Part print with two shaded views. Sizes in mm from the minimum x, y, z corner. A direction names the side the tool comes from. Round coordinates to 2 decimals unless told otherwise and drop trailing zeros. Loops run counter-clockwise (first coordinate to the right, second up) from the corner with the lowest first, then second, coordinate; pieces in that order, holes last.
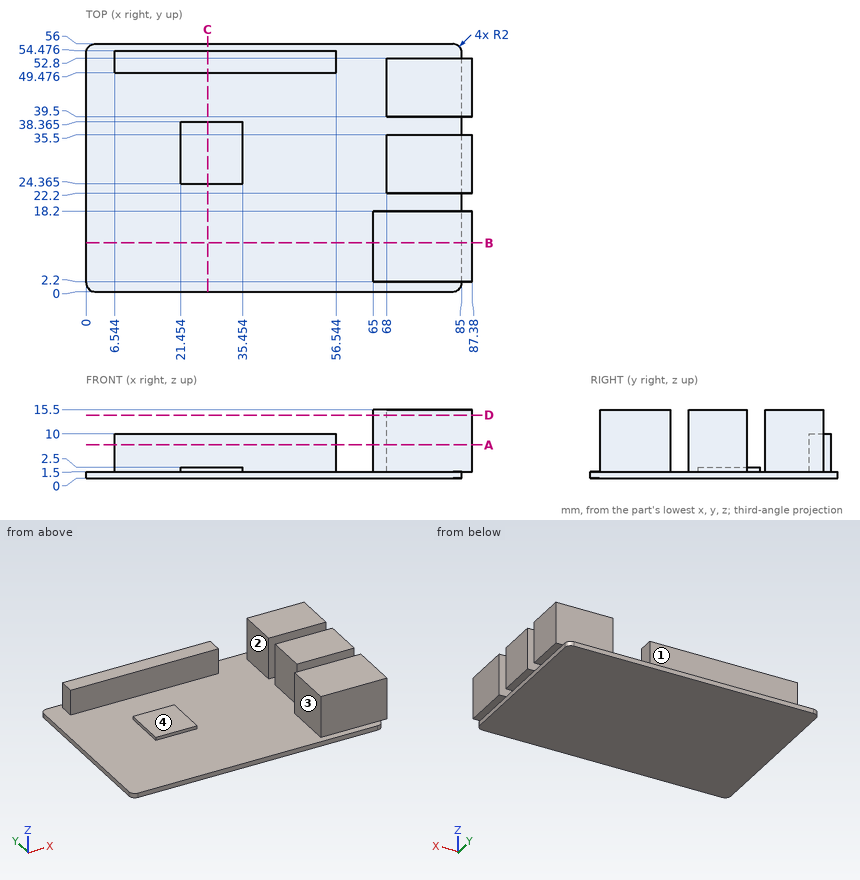
Item 1: Cut at A-A (z = 7.5). List the corners of the cut face in (x, y) (1 decimal).
Verdict:
outline: (6.5, 49.5) - (56.5, 49.5) - (56.5, 54.5) - (6.5, 54.5) - close; (65, 2.2) - (87.4, 2.2) - (87.4, 18.2) - (65, 18.2) - close; (68, 22.2) - (87.4, 22.2) - (87.4, 35.5) - (68, 35.5) - close; (68, 39.5) - (87.4, 39.5) - (87.4, 52.8) - (68, 52.8) - close
Item 2: Cut at C-C (x = 27.5). List the corners of the cut face in (y, z) (1 decimal).
Verdict:
outline: (0, 0) - (56, 0) - (56, 1.5) - (54.5, 1.5) - (54.5, 10) - (49.5, 10) - (49.5, 1.5) - (38.4, 1.5) - (38.4, 2.5) - (24.4, 2.5) - (24.4, 1.5) - (0, 1.5) - close
Item 3: Wall check: L1, parallel to Y at x = 73.5, z = 1.75; L2, parallel to X at y = 31, z = 1.75 (1 decimal); L3, parallel to Z at x = 48.5, y = 48.5. Give the ranges that are in metal, low to high.
Verdict:
L1: y = 2.2 to 18.2, 22.2 to 35.5, 39.5 to 52.8
L2: x = 21.5 to 35.5, 68 to 87.4
L3: z = 0 to 1.5
Item 4: Cut at D-D (z = 14.25). List the corners of the cut face in (x, y).
Verdict:
outline: (65, 2.2) - (87.38, 2.2) - (87.38, 18.2) - (65, 18.2) - close; (68, 22.2) - (87.38, 22.2) - (87.38, 35.5) - (68, 35.5) - close; (68, 39.5) - (87.38, 39.5) - (87.38, 52.8) - (68, 52.8) - close
Item 5: Flat gauge pins, fed straight in: P1, Ø6.5, axis at y = 45, z = 12, coming from the -X side; P2, Ø1.2, axis at y = 37, z = 1, coming from the +X side; P3, Ø4, axis at x = 33.5, y = 52, coming from the +Z side. Where does each tip first touch, or does it go through?
Verdict:
P1: stops at x = 68
P2: stops at x = 85
P3: stops at z = 10
Item 6: Cut at B-B (y = 11). List the corners of the cut face in (x, z), plus the area to 3 significant figures.
Verdict:
outline: (0, 0) - (85, 0) - (85, 1.5) - (87.38, 1.5) - (87.38, 15.5) - (65, 15.5) - (65, 1.5) - (0, 1.5) - close
area: 441 mm2
Item 7: 3-axis set-ups, long thin cutter, end or side, ignore diameter. For the marked faces 1, 2, 3 and 4: which of +Z, -Z, +X, -X, +Y, -Y reach the whole face in a straight line?
Verdict:
face 1: +Z, +X, -X, +Y
face 2: +Z, +Y
face 3: +Z, -X, +Y, -Y
face 4: +Z, -X, -Y
